Can you work these out from the model? Positions are in its coordinate system, mm. Face numbers are marked on the shaded views. A direction names the side the tool comes from. Coordinates: 2 decimals unless noted, no trailing zeros. Order: outer loops, then holes, each group sorted by start corner. A loop starts at its lowest first (then second) coordinate and runs counter-clockwise, first axis right, second up. Notation, with made-up numbers: (-18.75, 63.25) -> (6.25, 63.25) arc R27 cw to (6.25, 83.25) -> close; hole circle Ø4 at (-38.5, 22.5). An arc over 180 degrees is marked (long way). Answer in a Markdown table with one row per item.
```python
from build123d import *

# Parameters (mm, degrees)
F0_R     = 1.25
F0_W     = 12.5
F0_H     = 10
F0_W_2   = 19
F0_H_2   = 2
F0_W_3   = 3.25
F1_DEPTH = 6
F2_DEPTH = 21
F3_DEPTH = 13


with BuildPart() as f1:
    # F0 (on Top) → F1 (new body)
    with BuildSketch(Plane.XY):
        Polygon((9.5, 0), (9.5, 21), (-9.5, 21), (-9.5, 0), (-9.5, -11), (-6.25, -11), (6.25, -11), (9.5, -11), align=None)
        Polygon((14.5, -21), (14.5, 21), (9.5, 21), (9.5, 0), (9.5, -11), (9.5, -21), align=None)
        with Locations((11.25, -17.625)):
            Circle(F0_R, mode=Mode.SUBTRACT)
        with Locations((11.25, 17.625)):
            Circle(F0_R, mode=Mode.SUBTRACT)
        Polygon((-9.5, 0), (-9.5, 21), (-14.5, 21), (-14.5, -21), (-9.5, -21), (-9.5, -11), align=None)
        with Locations((-11.25, -17.625)):
            Circle(F0_R, mode=Mode.SUBTRACT)
        with Locations((-11.25, 17.625)):
            Circle(F0_R, mode=Mode.SUBTRACT)
        with Locations((0, -16)):
            Rectangle(F0_W, F0_H)
        Polygon((9.5, 21), (14.5, 21), (14.5, -21), (9.5, -21), (9.5, -23), (16.5, -23), (16.5, 23), (9.5, 23), align=None)
        Polygon((-14.5, 21), (-9.5, 21), (-9.5, 23), (-16.5, 23), (-16.5, -23), (-9.5, -23), (-9.5, -21), (-14.5, -21), align=None)
        with Locations((0, 22)):
            Rectangle(F0_W_2, F0_H_2)
        with Locations((7.875, -16)):
            Rectangle(F0_W_3, F0_H)
        with Locations((-7.875, -16)):
            Rectangle(F0_W_3, F0_H)
        with Locations((0, -22)):
            Rectangle(F0_W, F0_H_2)
        with Locations((7.875, -22)):
            Rectangle(F0_W_3, F0_H_2)
        with Locations((-7.875, -22)):
            Rectangle(F0_W_3, F0_H_2)
        with Locations((-11.25, 17.625)):
            Circle(F0_R)
        with Locations((11.25, 17.625)):
            Circle(F0_R)
        with Locations((-11.25, -17.625)):
            Circle(F0_R)
        with Locations((11.25, -17.625)):
            Circle(F0_R)
    extrude(amount=-F1_DEPTH)

    # F0 (on Top) → F2 (join)
    with BuildSketch(Plane.XY):
        Polygon((9.5, 21), (14.5, 21), (14.5, -21), (9.5, -21), (9.5, -23), (16.5, -23), (16.5, 23), (9.5, 23), align=None)
        Polygon((-14.5, 21), (-9.5, 21), (-9.5, 23), (-16.5, 23), (-16.5, -23), (-9.5, -23), (-9.5, -21), (-14.5, -21), align=None)
        with Locations((11.25, -17.625)):
            Circle(F0_R)
        with Locations((11.25, 17.625)):
            Circle(F0_R)
        with Locations((-11.25, 17.625)):
            Circle(F0_R)
        with Locations((-11.25, -17.625)):
            Circle(F0_R)
        with Locations((0, 22)):
            Rectangle(F0_W_2, F0_H_2)
        with Locations((-7.875, -22)):
            Rectangle(F0_W_3, F0_H_2)
        with Locations((7.875, -22)):
            Rectangle(F0_W_3, F0_H_2)
    extrude(amount=F2_DEPTH)

    # F0 (on Top) → F3 (join)
    with BuildSketch(Plane.XY):
        Polygon((14.5, -21), (14.5, 21), (9.5, 21), (9.5, 0), (9.5, -11), (9.5, -21), align=None)
        with Locations((11.25, -17.625)):
            Circle(F0_R, mode=Mode.SUBTRACT)
        with Locations((11.25, 17.625)):
            Circle(F0_R, mode=Mode.SUBTRACT)
        Polygon((-9.5, 0), (-9.5, 21), (-14.5, 21), (-14.5, -21), (-9.5, -21), (-9.5, -11), align=None)
        with Locations((-11.25, -17.625)):
            Circle(F0_R, mode=Mode.SUBTRACT)
        with Locations((-11.25, 17.625)):
            Circle(F0_R, mode=Mode.SUBTRACT)
        with Locations((-7.875, -16)):
            Rectangle(F0_W_3, F0_H)
        with Locations((-7.875, -22)):
            Rectangle(F0_W_3, F0_H_2)
        with Locations((7.875, -22)):
            Rectangle(F0_W_3, F0_H_2)
        with Locations((7.875, -16)):
            Rectangle(F0_W_3, F0_H)
    extrude(amount=F3_DEPTH)


solid = f1.part
```
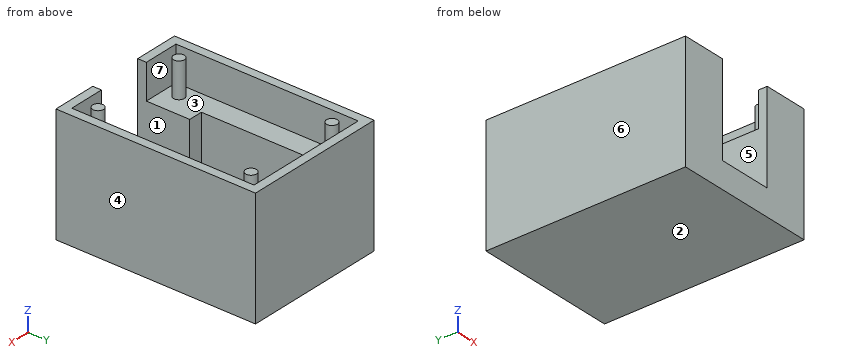
(1) Suppose I cut it at B-B (y = -12). Please give me the cut outline in (x, z), and give its area (4 significant figures).
Response values:
| item | result |
|---|---|
| outline | (-16.5, -6) -> (16.5, -6) -> (16.5, 21) -> (14.5, 21) -> (14.5, 13) -> (6.25, 13) -> (6.25, 0) -> (-6.25, 0) -> (-6.25, 13) -> (-14.5, 13) -> (-14.5, 21) -> (-16.5, 21) -> close |
| area | 496.5 mm2 |
(2) I need wall thicknesses on line 1 (Y direction, x = 12, z = 19.75) (3 decimals); line 2 (Y direction, x = -6.5, z = 5.75); line 3 (X direction, y = -5.5, z = 3.25). Which ranges of each line are inside material? Lowest first, please. Write a range as [from, to].
Response values:
| item | result |
|---|---|
| line 1 | [-23, -21], [-18.625, -16.625], [16.625, 18.625], [21, 23] |
| line 2 | [-23, -11], [21, 23] |
| line 3 | [-16.5, -9.5], [9.5, 16.5] |
(3) On a 3-axis mill with a long thin cutter (end or side, diameter ignored), from which of +Z, -Z, +X, -X, +Y, -Y can I reach the whole of each face in a straight line? I mean the marked faces 1, 2 and 3. Say none if no direction works.
Response values:
| item | result |
|---|---|
| face 1 | +Z, -Y |
| face 2 | -Z, +X, -X, +Y, -Y |
| face 3 | +Z |
(4) Suppose I cut it at C-C (z = 6). Please give me the cut outline in (x, y).
Response values:
| item | result |
|---|---|
| outline | (-16.5, -23) -> (-6.25, -23) -> (-6.25, -11) -> (-9.5, -11) -> (-9.5, 21) -> (9.5, 21) -> (9.5, -11) -> (6.25, -11) -> (6.25, -23) -> (16.5, -23) -> (16.5, 23) -> (-16.5, 23) -> close |
(5) Will these pins go through, and if not, where does the flat tip stop? pin 1 Ø8 at (x, y) = (3, -11) entering from +Z; pin 2 Ø5.5 at (x, y) = (-4.5, -8) entering from +Z.
Response values:
| item | result |
|---|---|
| pin 1 | z = 13 |
| pin 2 | z = 0 |
(6) We'd pull the mould along X, two halves only. Please class the marked faces 4, 5, 6 and 7: +X half, -X half, draft (parallel to the pull), parting line (faces both ways), or undercut.
Response values:
| item | result |
|---|---|
| face 4 | +X half |
| face 5 | undercut |
| face 6 | -X half |
| face 7 | undercut |
(7) Suppose I cut it at D-D (x = -11.25). Please give me the cut outline in (y, z) (3 decimals).
Response values:
| item | result |
|---|---|
| outline | (-23, -6) -> (23, -6) -> (23, 21) -> (21, 21) -> (21, 13) -> (18.875, 13) -> (18.875, 21) -> (16.375, 21) -> (16.375, 13) -> (-16.375, 13) -> (-16.375, 21) -> (-18.875, 21) -> (-18.875, 13) -> (-21, 13) -> (-21, 21) -> (-23, 21) -> close |
(8) Suppose I cut it at A-A (x = 7). Please give me the cut outline in (y, z), and give its area (3 significant figures).
Response values:
| item | result |
|---|---|
| outline | (-23, -6) -> (23, -6) -> (23, 21) -> (21, 21) -> (21, 0) -> (-11, 0) -> (-11, 13) -> (-21, 13) -> (-21, 21) -> (-23, 21) -> close |
| area | 490 mm2 |
